Geometry: final body of the model. Coordinates: model frame, mm. A direction names the side the tool comes from. Give positions to 0.01 mm unless a question says otherwise; leave off trailing zeros. Write each loop counter-clockwise with the first axis right and the second up, starting at its lowest first coordinate (ties: lowest second). Pieces come first, ordered by that corner, then holes. Notation, with made-up numbers: (58, -6) -> (107, -6) arc R19 ccw to (107, 31) -> close; hole circle Ø2 at (20.5, -12). An arc over 180 degrees is marked (long way). Answer as a JSON object with one key per item and string values.
from build123d import *

# Parameters (mm, degrees)
ESQUISSE1_R               = 10
BASE_DEPTH                = 5
BOSS_BALEINE_DEPTH        = 5
VIDE_BALEINE_DEPTH        = 3
REP_SUPPORT_BALEINE_COUNT = 5
CONGE_BALEINE_R           = 0.2


with BuildPart() as part:
    # Esquisse1 → BASE (new body)
    with BuildSketch(Plane(origin=(0, 0, 0), x_dir=(1, 0, 0), z_dir=(0, 1, 0))):
        with Locations(Location((0, 0, 0), (0, 0, 270))):
            Circle(ESQUISSE1_R)
    extrude(amount=-BASE_DEPTH)

    # Esquisse2 → BOSS - BALEINE (add)
    with BuildSketch(Plane(origin=(0, 0, 0), x_dir=(1, 0, 0), z_dir=(0, 1, 0))):
        with BuildLine():
            ThreePointArc((9.38083152, -1.5), (9.486684928, -0.502801231), (9.486832981, 0.5))
            Line((9.486832981, 0.5), (17.38083152, 0.5))
            Line((17.38083152, 0.5), (17.38083152, -1.5))
            Line((17.38083152, -1.5), (9.38083152, -1.5))
        make_face()
    boss_baleine = extrude(amount=-BOSS_BALEINE_DEPTH)

    # Esquisse3 → VIDE - BALEINE (cut)
    with BuildSketch(Plane.XY.offset(1.5)):
        with BuildLine():
            Line((13.88083152, 0), (13.820171348, -1.439339828))
            ThreePointArc((13.820171348, -1.439339828), (14.88083152, -4), (15.941491691, -1.439339828))
            Line((15.941491691, -1.439339828), (15.88083152, 0))
            Line((15.88083152, 0), (13.88083152, 0))
        make_face()
    vide_baleine = extrude(amount=-VIDE_BALEINE_DEPTH, mode=Mode.SUBTRACT)

    # REP - SUPPORT BALEINE: BOSS - BALEINE, VIDE - BALEINE ×5 about axis
    rep_support_baleine_axis = Axis((0, 0, 0), (0, 1, 0))
    add([boss_baleine.rotate(rep_support_baleine_axis, i * 360 / REP_SUPPORT_BALEINE_COUNT) for i in range(1, REP_SUPPORT_BALEINE_COUNT)])
    add([vide_baleine.rotate(rep_support_baleine_axis, i * 360 / REP_SUPPORT_BALEINE_COUNT) for i in range(1, REP_SUPPORT_BALEINE_COUNT)], mode=Mode.SUBTRACT)

    # CONGE BALEINE
    conge_baleine_edges = [part.edges().sort_by_distance(p)[0] for p in [
        (4.764941094, 0, -13.046946771),
        (5.382975083, 0, -14.949059804),
        (-10.935935969, 0, -8.563456554),
        (-12.553969958, 0, -9.739027059),
        (-11.523721222, 0, 7.75443956),
        (-13.14175521, 0, 8.930010064),
        (3.813884577, 0, 13.355963766),
        (4.431918566, 0, 15.258076798),
        (13.88083152, 0, 0.5),
        (15.88083152, 0, 0.5),
    ]]
    fillet(conge_baleine_edges, radius=CONGE_BALEINE_R)


solid = part.part
Q1. Cut plane C-C (x = -2). Return the cut outline in (y, z).
Values:
{"outline": "(-5, -9.8) -> (0, -9.8) -> (0, 9.8) -> (-5, 9.8) -> close"}
Q2. Mould query, pull axis Y, two halves, no side actions, for faces 6 (the flat face through (-11.504, -0.815, 7.723)), 7 (the flat face through (6, 0, -16)), 8 (the cylindrical face through (-9.983, -2.465, -0.576)). Classes: pulls with the +Y half, pulls with the -Y half, needs draft (parallel to the pull), parting line crosses it, or undercut.
Values:
{"face 6": "undercut", "face 7": "pulls with the +Y half", "face 8": "needs draft"}
Q3. Cut plane B-B (z = -3.5). Return the cut outline in (x, y).
Values:
{"outline": "(-9.37, -5) -> (9.37, -5) -> (9.37, 0) -> (-9.37, 0) -> close"}
Q4. Material intervals for L1, parallel to X at y = -2.5, z = 0.4; L2, parallel to Z at x = -13, y = -0.75; L3, parallel to X at y = -1, z = -11, sorted ascending. Write a range as from..to.
Values:
{"L1": "-9.99..13.38, 16.38..17.38", "L2": "-11.3..-9.18, 9.18..10.06", "L3": "-13.49..-12.59, 3.05..5.15"}
Q5. Set-up query: faces 1 (the flat face through (13, -2, 1.5)), 2 (the flat face through (3.79, -0.815, 13.328)), 3 (the cylindrical face through (-12.3, -4, 8.3)), 4 (the cylindrical face through (8, -2, 6)), 5 (the flat face through (13.846, -0.815, 0.514)). Return all of +Z, -Z, +X, -X, +Y, -Y with unobstructed straight access to the full face (end or side cutting, diameter ignored); none if empty.
Values:
{"face 1": "+Z, +X, +Y, -Y", "face 2": "+X", "face 3": "none", "face 4": "+X, +Y, -Y", "face 5": "+Z, -Z"}
Q6. Cut plane A-A (y = -3.05). State how many separate pieces and enclosed holes the cut face has, and give its area (3 significant figures).
Values:
{"separate pieces": "6", "enclosed holes": "0", "area": "360 mm²"}
Q7. First-contact query: P1, Ø1.5, axis at x = 14, y = -3, coming from the -Z side; P2, Ø1.5, axis at y = -1, z = 10.5, coming from the +X side; P3, Ø1.5, axis at y = -4.5, z = 0, coming from the -X side. Flat tips, straight axial feed; report the tip coordinate or a pass-through.
Values:
{"P1": "z = -0.5", "P2": "x = 4.18", "P3": "x = -10"}
